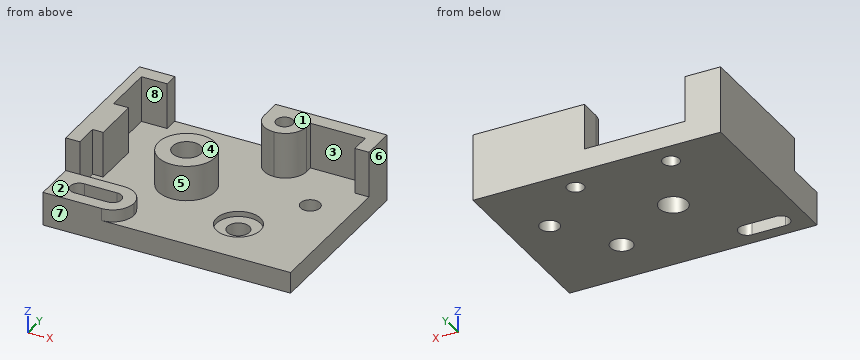
```python
from build123d import *

# Parameters (mm, degrees)
F0_W      = 140
F0_H      = 38
F1_DEPTH  = 102
F2_R      = 4.75
F3_DEPTH  = 40
F4_R      = 8
F5_DEPTH  = 40
F6_R      = 6.25
F7_DEPTH  = 40
F8_R      = 5.5
F9_DEPTH  = 40
F10_W     = 140
F10_H     = 26
F11_DEPTH = 102
F12_R     = 16
F13_DEPTH = 26
F14_R     = 8
F15_DEPTH = 26
F16_W     = 45
F16_H     = 24
F17_DEPTH = 7
F18_R     = 12
F19_R     = 11.99999
F20_W     = 20
F20_H     = 78
F21_DEPTH = 26
F22_W     = 63
F22_H     = 24
F23_DEPTH = 26
F24_R     = 4.75
F25_DEPTH = 38
F26_R     = 12
F27_R     = 5
F28_DEPTH = 40
F30_DEPTH = 40
F31_W     = 19
F31_H     = 5
F32_DEPTH = 40
F33_W     = 31
F33_H     = 16
F34_DEPTH = 26
F35_R     = 11.99999
F36_W     = 8
F36_H     = 5
F37_DEPTH = 26
F38_R     = 16
F39_DEPTH = 6
F40_W     = 6
F40_H     = 74.1499609053
F41_DEPTH = 26
F42_W     = 6
F42_H     = 4
F43_DEPTH = 26
F44_W     = 6
F44_H     = 13.5
F45_DEPTH = 26
F46_W     = 8.5837110281
F46_H     = 29.5
F47_DEPTH = 26
F48_W     = 6
F48_H     = 0.1499609053
F49_DEPTH = 26
F50_R     = 12.5
F51_DEPTH = 3


# Not quite as in the source:
# - a fillet or chamfer is up to 0.001 mm smaller than in the source, because OpenCascade refuses the exact size


with BuildPart() as f1:
    # F0 (on Front) → F1 (new body)
    with BuildSketch(Plane.XZ):
        with Locations((70, 19)):
            Rectangle(F0_W, F0_H)
    extrude(amount=F1_DEPTH)

    # F2 (on face) → F3 (cut)
    with BuildSketch(Plane.XY.offset(38)):
        with Locations((35, -13)):
            Circle(F2_R)
        with Locations((89, -13)):
            Circle(F2_R)
    extrude(amount=-F3_DEPTH, mode=Mode.SUBTRACT)

    # F4 (on face) → F5 (cut)
    with BuildSketch(Plane.XY.offset(38)):
        with Locations((54, -51)):
            Circle(F4_R)
    extrude(amount=-F5_DEPTH, mode=Mode.SUBTRACT)

    # F6 (on face) → F7 (cut)
    with BuildSketch(Plane.XY.offset(38)):
        with Locations((95, -73)):
            Circle(F6_R)
    extrude(amount=-F7_DEPTH, mode=Mode.SUBTRACT)

    # F8 (on face) → F9 (cut)
    with BuildSketch(Plane.XY.offset(38)):
        with Locations((118, -40)):
            Circle(F8_R)
    extrude(amount=-F9_DEPTH, mode=Mode.SUBTRACT)

    # F10 (on face) → F11 (cut)
    with BuildSketch(Plane.XZ.offset(102)):
        with Locations((70, 25)):
            Rectangle(F10_W, F10_H)
    extrude(amount=-F11_DEPTH, mode=Mode.SUBTRACT)

    # F12 (on face) → F13 (join)
    with BuildSketch(Plane.XY.offset(12)):
        with Locations((54, -51)):
            Circle(F12_R)
    extrude(amount=F13_DEPTH)

    # F14 (on face) → F15 (cut)
    with BuildSketch(Plane.XY.offset(38)):
        with Locations((54, -51)):
            Circle(F14_R)
    extrude(amount=-F15_DEPTH, mode=Mode.SUBTRACT)

    # F16 (on face) → F17 (join)
    with BuildSketch(Plane.XY.offset(12)):
        with Locations((22.5, -90)):
            Rectangle(F16_W, F16_H)
    extrude(amount=F17_DEPTH)

    # F18
    f18_edges = [f1.edges().sort_by_distance(p)[0] for p in [
        (45, -78, 15.5),
    ]]
    fillet(f18_edges, radius=F18_R)

    # F19 (radius 12 in the source; OpenCascade refuses exactly that, so slightly less here)
    f19_edges = [f1.edges().sort_by_distance(p)[0] for p in [
        (45, -102, 15.5),
    ]]
    fillet(f19_edges, radius=F19_R)

    # F20 (on face) → F21 (join)
    with BuildSketch(Plane.XY.offset(12)):
        with Locations((10, -39)):
            Rectangle(F20_W, F20_H)
    extrude(amount=F21_DEPTH)

    # F22 (on face) → F23 (join)
    with BuildSketch(Plane.XY.offset(12)):
        with Locations((108.5, -12)):
            Rectangle(F22_W, F22_H)
    extrude(amount=F23_DEPTH)

    # F24 (on face) → F25 (cut)
    with BuildSketch(Plane(origin=(0, 0, 0), x_dir=(1, 0, 0), z_dir=(0, 0, -1))):
        with Locations((89, 13)):
            Circle(F24_R)
    extrude(amount=-F25_DEPTH, mode=Mode.SUBTRACT)

    # F26
    f26_edges = [f1.edges().sort_by_distance(p)[0] for p in [
        (77, -24, 25),
    ]]
    fillet(f26_edges, radius=F26_R)

    # F27 (on face) → F28 (cut)
    with BuildSketch(Plane.XY.offset(19)):
        with Locations((14, -90)):
            Circle(F27_R)
        with Locations((33, -90)):
            Circle(F27_R)
    extrude(amount=-F28_DEPTH, mode=Mode.SUBTRACT)

    # F29 (on face) → F30 (cut)
    with BuildSketch(Plane.XY.offset(19)):
        with BuildLine():
            ThreePointArc((14.2498681067, -85.00624731), (17.6227986788, -86.5539399696), (19, -90))
            Line((19, -90), (28, -90))
            ThreePointArc((28, -90), (29.3772013212, -86.5539399696), (32.7501318933, -85.00624731))
            Line((32.7501318933, -85.00624731), (14.2498681067, -85.00624731))
        make_face()
    extrude(amount=-F30_DEPTH, mode=Mode.SUBTRACT)

    # F31 (on face) → F32 (cut)
    with BuildSketch(Plane.XY.offset(19)):
        with Locations((23.5, -92.5)):
            Rectangle(F31_W, F31_H)
    extrude(amount=-F32_DEPTH, mode=Mode.SUBTRACT)

    # F33 (on face) → F34 (cut)
    with BuildSketch(Plane.XY.offset(38)):
        with Locations((116.5, -16)):
            Rectangle(F33_W, F33_H)
    extrude(amount=-F34_DEPTH, mode=Mode.SUBTRACT)

    # F35 (radius 12 in the source; OpenCascade refuses exactly that, so slightly less here)
    f35_edges = [f1.edges().sort_by_distance(p)[0] for p in [
        (101, -24, 25),
    ]]
    fillet(f35_edges, radius=F35_R)

    # F36 (on face) → F37 (cut)
    with BuildSketch(Plane.XY.offset(38)):
        with Locations((136, -21.5)):
            Rectangle(F36_W, F36_H)
    extrude(amount=-F37_DEPTH, mode=Mode.SUBTRACT)

    # F38 (on face) → F39 (cut)
    with BuildSketch(Plane.XY.offset(38)):
        with Locations((54, -51)):
            Circle(F38_R)
    extrude(amount=-F39_DEPTH, mode=Mode.SUBTRACT)

    # F40 (on face) → F41 (cut)
    with BuildSketch(Plane.XY.offset(38)):
        with Locations((17, -40.9250195473)):
            Rectangle(F40_W, F40_H)
    extrude(amount=-F41_DEPTH, mode=Mode.SUBTRACT)

    # F42 (on face) → F43 (join)
    with BuildSketch(Plane.XY.offset(12)):
        with Locations((17, -5.8500390947)):
            Rectangle(F42_W, F42_H)
    extrude(amount=F43_DEPTH)

    # F44 (on face) → F45 (cut)
    with BuildSketch(Plane.XY.offset(38)):
        with Locations((11, -71.25)):
            Rectangle(F44_W, F44_H)
    extrude(amount=-F45_DEPTH, mode=Mode.SUBTRACT)

    # F46 (on face) → F47 (cut)
    with BuildSketch(Plane.XY.offset(38)):
        with Locations((9.708144486, -22.75)):
            Rectangle(F46_W, F46_H)
    extrude(amount=-F47_DEPTH, mode=Mode.SUBTRACT)

    # F48 (on face) → F49 (join)
    with BuildSketch(Plane.XY.offset(38)):
        with Locations((17, -7.9250195473)):
            Rectangle(F48_W, F48_H)
    extrude(amount=-F49_DEPTH)

    # F50 (on face) → F51 (cut)
    with BuildSketch(Plane.XY.offset(12)):
        with Locations((95, -73)):
            Circle(F50_R)
    extrude(amount=-F51_DEPTH, mode=Mode.SUBTRACT)


solid = f1.part
```
The listing builds one solid part. Answer for the finished solid, in the listing's coordinates (mm). Face numbers are marked on the shaded views. A direction names the side the tool comes from. Give positions to 0.01 mm unless a question says otherwise; leave off trailing zeros. Loops run counter-clockwise (first coordinate to the right, second up) from the corner with the lowest first, then second, coordinate; pieces in that order, holes last. Notation, with made-up numbers: M 5.5,24.5 L 40.5,24.5 A24 ccw 40.5,52.5 Z; hole C 84.25,14 d4. An arc over 180 degrees is marked long. One line per item, written item: value.
Q1. A cutting plane is placed at A-A on x = 54. Determine the outline of the cut face in (y, z).
Working result:
outline: M -102,0 L -59,0 L -59,32 L -67,32 L -67,12 L -102,12 Z; M -43,0 L 0,0 L 0,12 L -35,12 L -35,32 L -43,32 Z
Q2. Determine the mould class of the marked faces 6, 7 and 8 for opening direction X: +X half, -X half, draft (parallel to the pull), parting line (faces both ways), or undercut.
Working result:
face 6: +X half
face 7: draft
face 8: undercut
Q3. For the marked faces 1, 2, 3, 4 and 5, determine the directions among +Z, -Z, +X, -X, +Y, -Y from which every point of the face is accessible in a straight line to the end or side of a thin tool.
Working result:
face 1: +Z, +X, -X, +Y, -Y
face 2: +Z, +X, -X, -Y
face 3: +Z, -Y
face 4: +Z, +X, +Y, -Y
face 5: +Z
Q4. Flat-ended cylindrical pins translate along their axes: P1, Ø13, axis at x = 113, z = 23, coming from the -Y side; P2, Ø6, axis at x = 65, y = -85.5, coming from the -Z side; P3, Ø12.5, axis at x = 35, y = -13, coming from the +Z side; P4, Ø4, axis at x = 99, z = 32, coming from the -Y side. Find the tip coordinate at first contact, or state that the pin passes through.
Working result:
P1: stops at y = -8
P2: stops at z = 0
P3: stops at z = 12
P4: stops at y = -20.94
Q5. A cutting plane is placed at C-C on x = 87. Determine the outline of the cut face in (y, z).
Working result:
outline: M -102,0 L -17.31,0 L -17.31,38 L -23.83,38 L -23.83,12 L -63.4,12 L -63.4,9 L -82.6,9 L -82.6,12 L -102,12 Z; M -8.69,0 L 0,0 L 0,38 L -8.69,38 Z
Q6. A cutting plane is placed at B-B on y = -51. Determine the outline of the cut face in (x, z), then the cut area to 3 significant figures.
Working result:
outline: M 0,0 L 46,0 L 46,32 L 38,32 L 38,12 L 14,12 L 14,38 L 0,38 Z; M 62,0 L 140,0 L 140,12 L 70,12 L 70,32 L 62,32 Z
area: 2,170 mm^2
Q7. A cutting plane is placed at D-D on x = 110.5. Determine the outline of the cut face in (y, z), then the cut area to 3 significant figures.
Working result:
outline: M -102,0 L 0,0 L 0,38 L -8,38 L -8,12 L -102,12 Z
area: 1,430 mm^2
Q8. Find the intervals of material crossed by line 1 (X direction, y = -13, z = 21); line 2 (Y direction, x = 35, z = 5.5); line 3 (Y direction, x = 95, z = 10), in increasing order. Write a range as from..to.
Working result:
line 1: x = 0..5.42, 77.04..84.25, 93.75..100.96, 132..140
line 2: y = -102..-94.58, -85.42..-17.75, -8.25..0
line 3: y = -102..-85.5, -60.5..0
